from build123d import *

# Parameters (mm, degrees)
SKETCH_R  = 12.7
PAD_DEPTH = 9.525


with BuildPart() as part:
    # Sketch → Pad (new body)
    with BuildSketch(Plane.XZ):
        Polygon((-60.157258, 57.66002), (31.155391, 57.66002), (56.555391, 32.26002), (56.555391, 19.56002), (31.155391, -5.83998), (-85.557258, -5.83998), (-85.557258, 32.26002), align=None)
        with Locations((-53.807258, 27.51022)):
            Circle(SKETCH_R, mode=Mode.SUBTRACT)
        with Locations((22.392742, 27.51022)):
            Circle(SKETCH_R, mode=Mode.SUBTRACT)
    extrude(amount=PAD_DEPTH)


solid = part.part
Source: CAD feature listing. Evaluate the final solid. Frame: model axes, mm. Give positions to 0.01 mm unless a question says otherwise; leave off trailing zeros. Order: outer loops, then holes, each group sorted by start corner. A loop starts at its lowest first (then second) coordinate and runs counter-clockwise, first axis right, second up. Notation, with made-up numbers: (73, 46.25) -> (121, 46.25) arc R24 ccw to (121, 65.25) -> close; hole circle Ø8 at (71, -28.5). An arc over 180 degrees is marked (long way). Use a Markdown table: item, result.
1) Ray query, line 1 along X through (y, z) = (-5, 30.5); line 2 along X through (y, z) = (-7, 21); line 3 along Z through (x, y) = (23, -3.75). Return the intervals inside material, ascending. Write a range as [from, to].
Answer list:
| item | result |
|---|---|
| line 1 | [-85.56, -66.15], [-41.46, 10.05], [34.74, 56.56] |
| line 2 | [-85.56, -64.71], [-42.9, 11.49], [33.3, 56.56] |
| line 3 | [-5.84, 14.82], [40.2, 57.66] |
2) Section query A-A, the plane y = -7.5. Return the cut outline in (x, z).
Answer list:
| item | result |
|---|---|
| outline | (-85.56, -5.84) -> (31.16, -5.84) -> (56.56, 19.56) -> (56.56, 32.26) -> (31.16, 57.66) -> (-60.16, 57.66) -> (-85.56, 32.26) -> close; hole circle Ø25.4 at (-53.81, 27.51); hole circle Ø25.4 at (22.39, 27.51) |
3) Section query C-C, the plane z = 26. Return the cut outline in (x, y) (3 decimals), then the cut area to 3 significant figures.
Answer list:
| item | result |
|---|---|
| outline | (-85.557, -9.525) -> (-66.417, -9.525) -> (-66.417, 0) -> (-85.557, 0) -> close; (-41.197, -9.525) -> (9.783, -9.525) -> (9.783, 0) -> (-41.197, 0) -> close; (35.003, -9.525) -> (56.555, -9.525) -> (56.555, 0) -> (35.003, 0) -> close |
| area | 873 mm² |
4) Mould query, pull axis X, two halves, no side actions, for faces 1 (the cylindrical face through (-47.95, -4.7, 16.24)), 2 (the flat face through (-15, -5, 57.66)), 3 (the flat face through (56.555, -5, 26)). Classes: +X half, -X half, draft (parallel to the pull), parting line (faces both ways), or undercut.
Answer list:
| item | result |
|---|---|
| face 1 | undercut |
| face 2 | draft |
| face 3 | +X half |
5) Section query D-D, the plane x = -46.5. Return the cut outline in (y, z) (3 decimals).
Answer list:
| item | result |
|---|---|
| outline | (-9.525, -5.84) -> (0, -5.84) -> (0, 17.123) -> (-9.525, 17.123) -> close; (-9.525, 37.897) -> (0, 37.897) -> (0, 57.66) -> (-9.525, 57.66) -> close |
6) Contact query for flat-ended pins moving along their axis: P1, Ø6, axis at x = -44, z = 49.5, coming from the +Y side; P2, Ø1, axis at y = -3.5, z = 3, coming from the +X side. Output: stop coordinate, or through.
Answer list:
| item | result |
|---|---|
| P1 | y = 0 |
| P2 | x = 40.5 |
7) Section query B-B, the plane x = -65. Return the cut outline in (y, z) (3 decimals).
Answer list:
| item | result |
|---|---|
| outline | (-9.525, -5.84) -> (0, -5.84) -> (0, 21.509) -> (-9.525, 21.509) -> close; (-9.525, 33.511) -> (0, 33.511) -> (0, 52.817) -> (-9.525, 52.817) -> close |
